from build123d import *

# Parameters (mm, degrees)
F2_D     = 4
F3_D     = 4
F4_D     = 4
F4_DEPTH = 150
F5_D     = 4
F5_DEPTH = 150


with BuildPart() as f1:
    # F0 (on Front) → F1 (revolve)
    with BuildSketch(Plane.XZ):
        with BuildLine():
            Line((7.5, -75), (8.5, -75))
            Line((8.5, -75), (8.5, 75))
            Line((8.5, 75), (7.5, 75))
            Line((7.5, 75), (7.5, 105))
            Line((7.5, 105), (0, 105))
            Line((0, 105), (0, 104))
            ThreePointArc((0, 104), (3, 101), (0, 98))
            Line((0, 98), (0, -98))
            ThreePointArc((0, -98), (3, -101), (0, -104))
            Line((0, -104), (0, -105))
            Line((0, -105), (7.5, -105))
            Line((7.5, -105), (7.5, -75))
        make_face()
    revolve(axis=Axis((0, 0, 64.221174), (0, 0, 1)))

    # F2 (through all)
    with Locations(Plane.XZ):
        with Locations((0, 101)):
            Hole(F2_D / 2)

    # F3 (through all)
    with Locations(Plane(origin=(0, 0, 0), x_dir=(1, 0, 0), z_dir=(0, 1, 0))):
        with Locations((0, 101)):
            Hole(F3_D / 2)

    # F4
    with Locations(Plane(origin=(0, 0, 0), x_dir=(1, 0, 0), z_dir=(0, 1, 0))):
        with Locations((0, -101)):
            Hole(F4_D / 2, depth=F4_DEPTH)

    # F5
    with Locations(Plane.XZ):
        with Locations((0, -101)):
            Hole(F5_D / 2, depth=F5_DEPTH)


solid = f1.part
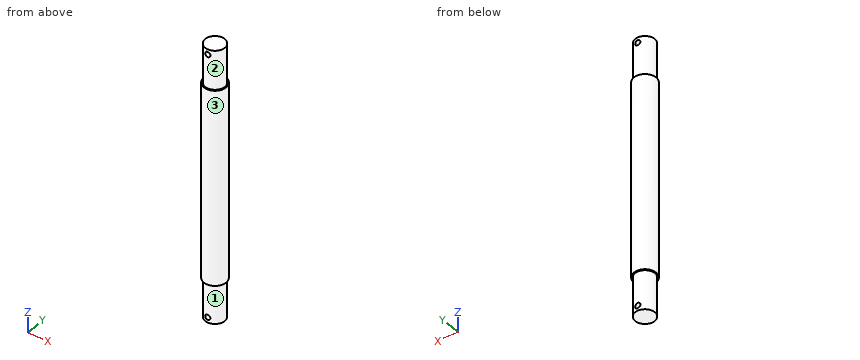
Could you check a few things on this model? Use its own coordinates, in mm. Face numbers are marked on the shaded views. A direction names the side the tool comes from. Coordinates: 2 decimals unless noted, no trailing zeros. Order: outer loops, then holes, each group sorted by start corner. A loop starts at its lowest first (then second) coordinate and runs counter-clockwise, first axis right, second up.
Q1. Suppose I cut it at A-A on y = 0. Please give me the cut outline in (x, z), and give its area (3 significant figures).
Q2. Suppose I cut it at C-C on z = 101. Please give me the cut outline in (x, y).
Q3. Please list where these lines run through material, in increasing order: L1, parallel to Z at x = 0, y = -5.4; L2, parallel to Z at x = 1, y = -0.5; L3, parallel to Z at x = 5.25, y = -6.
Q4. Suppose I cut it at B-B on x = 0. Please give me the cut outline in (y, z).
Q5. Which directions (+Z, -Z, +X, -X, +Y, -Y) give clear straight access to the entire face, cutting with the end or side of a thin tool? Please do the marked faces 1, 2 and 3.
Q6. Suppose I cut it at D-D on z = -10. Please give me the cut outline in (x, y), and give its area (3 significant figures).
Q7. Will these pins go through, and if not, where does the flat tip stop? pin 1 (1.5 mm diameter, centred on x = 0.5, z = 70, fed in from -Y); pin 2 (4 mm diameter, centred on x = -5.5, z = -40.5, fed in from -Y); pin 3 (4.5 mm diameter, centred on x = 0, z = -101, fed in from -Y); pin 4 (3 mm diameter, centred on x = 0, z = -101, fed in from +Y).
Answer:
1. outline: (-8.5, -75) - (-7.5, -75) - (-7.5, -105) - (7.5, -105) - (7.5, -75) - (8.5, -75) - (8.5, 75) - (7.5, 75) - (7.5, 105) - (-7.5, 105) - (-7.5, 75) - (-8.5, 75) - close; hole circle Ø6 at (0, -101); hole circle Ø6 at (0, 101)
1. area: 3,390 mm2
2. outline: (-2, -7.23) - (-2, -2.24) arc R3 cw to (-2, 2.24) - (-2, 7.23) arc R7.5 ccw to start; (2, -7.23) arc R7.5 ccw to (2, 7.23) - (2, 2.24) arc R3 cw to (2, -2.24) - close
3. L1: z = -105 to -103, -99 to 99, 103 to 105
3. L2: z = -105 to -103.78, -98.22 to 98.22, 103.78 to 105
3. L3: z = -75 to 75
4. outline: (-8.5, -75) - (-7.5, -75) - (-7.5, -99) - (-2.24, -99) arc R3 cw to (2.24, -99) - (7.5, -99) - (7.5, -75) - (8.5, -75) - (8.5, 75) - (7.5, 75) - (7.5, 99) - (2.24, 99) arc R3 cw to (-2.24, 99) - (-7.5, 99) - (-7.5, 75) - (-8.5, 75) - close; (-7.5, -105) - (7.5, -105) - (7.5, -103) - (2.24, -103) arc R3 cw to (-2.24, -103) - (-7.5, -103) - close; (-7.5, 103) - (-2.24, 103) arc R3 cw to (2.24, 103) - (7.5, 103) - (7.5, 105) - (-7.5, 105) - close
5. face 1: -Z
5. face 2: +Z
5. face 3: +Z, -Z
6. outline: circle Ø17 at (0, 0)
6. area: 227 mm2
7. pin 1: stops at y = -8.5
7. pin 2: stops at y = -7.75
7. pin 3: stops at y = -7.5
7. pin 4: passes through
